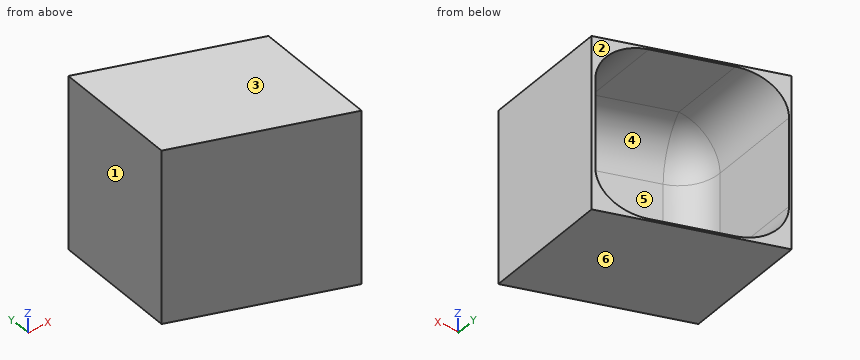
from build123d import *

# Parameters (mm, degrees)
BOSS_EXTRUDE1_DEPTH = 38.1
SHELL1_START        = -37.25333418
SHELL1_DEPTH        = 74.50666836
FILLET1_R           = 17.78


# Read off the part's stored shape, not the designer's step: Shell1
with BuildPart() as part:
    # Sketch1 → Boss-Extrude1 (new, symmetric)
    with BuildSketch(Plane.XY):
        Polygon((-33.198119966, 25.4), (-33.198119966, -25.4), (33.198119966, -50.887128572), (33.198119966, -0.087128572), align=None)
    extrude(amount=BOSS_EXTRUDE1_DEPTH, both=True)

    # Shell1 outline → Shell1 (cut)
    with BuildSketch(Plane.XY.offset(SHELL1_START)):
        Polygon((-32.351454146, 25.074995442), (-32.351454146, -24.818102704), (31.928119966, -49.492719393), (31.928119966, 0.400378753), align=None)
    extrude(amount=SHELL1_DEPTH, mode=Mode.SUBTRACT)

    # Fillet1
    fillet1_edges = [part.edges().sort_by_distance(p)[0] for p in [
        (-32.351454146, 0.128446369, -37.25333418),
        (-0.21166709, -37.155411048, -37.25333418),
        (-32.351454146, -24.818102704, 0),
        (31.928119966, -24.54617032, -37.25333418),
        (31.928119966, -49.492719393, 0),
        (-32.351454146, 0.128446369, 37.25333418),
        (-0.21166709, -37.155411048, 37.25333418),
        (31.928119966, -24.54617032, 37.25333418),
    ]]
    fillet(fillet1_edges, radius=FILLET1_R)


solid = part.part
Could you check a few things on this model? Use its own coordinates, in mm. Face numbers are marked on the shaded views. A direction names the side the tool comes from. Give positions to 0.01 mm unless a question says otherwise; leave off trailing zeros. Order: outer loops, then holes, each group sorted by start corner. A loop starts at its lowest first (then second) coordinate and runs counter-clockwise, first axis right, second up. Notation, with made-up numbers: (16.25, 52) -> (74.25, 52) arc R28 ccw to (74.25, 87) -> close; hole circle Ø1 at (31, -35.75). An arc over 180 degrees is marked (long way). Answer in a Markdown table with one row per item. Add a question column.
Item 1: Imagine slicing it at B-B (z = -1). List the corners of the cut face in (x, y) for me (3 decimals).
Item 2: We'd pull the mould along X, two halves only. Please class the marked faces 1, 2, 3 and 4: pulls with the +X half, pulls with the -X half, needs draft (parallel to the pull), parting line crosses it, or undercut.
Item 3: Please list where these lines run through material, in increasing order: probe 1 along Z at (x, y) = (-11.5, -8.5); probe 2 along X at (y, z) = (-13, 4); probe 3 along X at (y, z) = (22, -17).
Item 4: Imagine slicing it at C-C (x = 17). List the corners of the cut face in (y, z) for me.
Item 5: I'm going to push flat-ended pins straight in: P1, Ø5, axis at x = 6.5, z = 3.5, coming from the -Y side; P2, Ø3, axis at x = 3.5, z = -29, coming from the -Y side; P3, Ø4, axis at x = 18, z = 2.5, coming from the +Y side. Where does each tip first touch, or does it pass through?
Item 6: Imagine slicing it at A-A (y = -2.5). List the corners of the cut face in (x, z) for me.
Item 7: For the marked faces 5 and 6, which set-ups out of +Z, -Z, +X, -X, +Y, -Y let a thin tool reach every point of the face, with its end or its side?
Result:
| question | item | result |
|---|---|---|
| 1 | outline | (-33.198, -25.4) -> (33.198, -50.887) -> (33.198, -0.087) -> (31.928, 0.4) -> (31.928, -23.623) arc R17.78 cw to (7.776, -40.222) -> (-20.943, -29.197) arc R17.78 cw to (-32.351, -12.598) -> (-32.351, 25.075) -> (-33.198, 25.4) -> close |
| 2 | face 1 | pulls with the -X half |
| 2 | face 2 | pulls with the +X half |
| 2 | face 3 | needs draft |
| 2 | face 4 | undercut |
| 3 | probe 1 | -38.1 to -37.25, 37.25 to 38.1 |
| 3 | probe 2 | -33.2 to -32.35, 31.93 to 33.2 |
| 3 | probe 3 | -33.2 to -32.35 |
| 4 | outline | (-44.67, -38.1) -> (6.13, -38.1) -> (6.13, -37.02) -> (-23.62, -37.02) arc R17.55 cw to (-41.17, -19.47) -> (-41.17, 19.47) arc R17.55 cw to (-23.62, 37.02) -> (6.13, 37.02) -> (6.13, 38.1) -> (-44.67, 38.1) -> close |
| 5 | P1 | y = -41.6 |
| 5 | P2 | y = -40.06 |
| 5 | P3 | y = -40.41 |
| 6 | outline | (-33.2, -38.1) -> (33.2, -38.1) -> (33.2, 38.1) -> (-33.2, 38.1) -> close; hole (-32.35, -19.47) arc R17.78 ccw to (-14.57, -37.25) -> (14.15, -37.25) arc R17.78 ccw to (31.93, -19.47) -> (31.93, 19.47) arc R17.78 ccw to (14.15, 37.25) -> (-14.57, 37.25) arc R17.78 ccw to (-32.35, 19.47) -> close |
| 7 | face 5 | +Y |
| 7 | face 6 | -Z, +X, -X, +Y, -Y |
